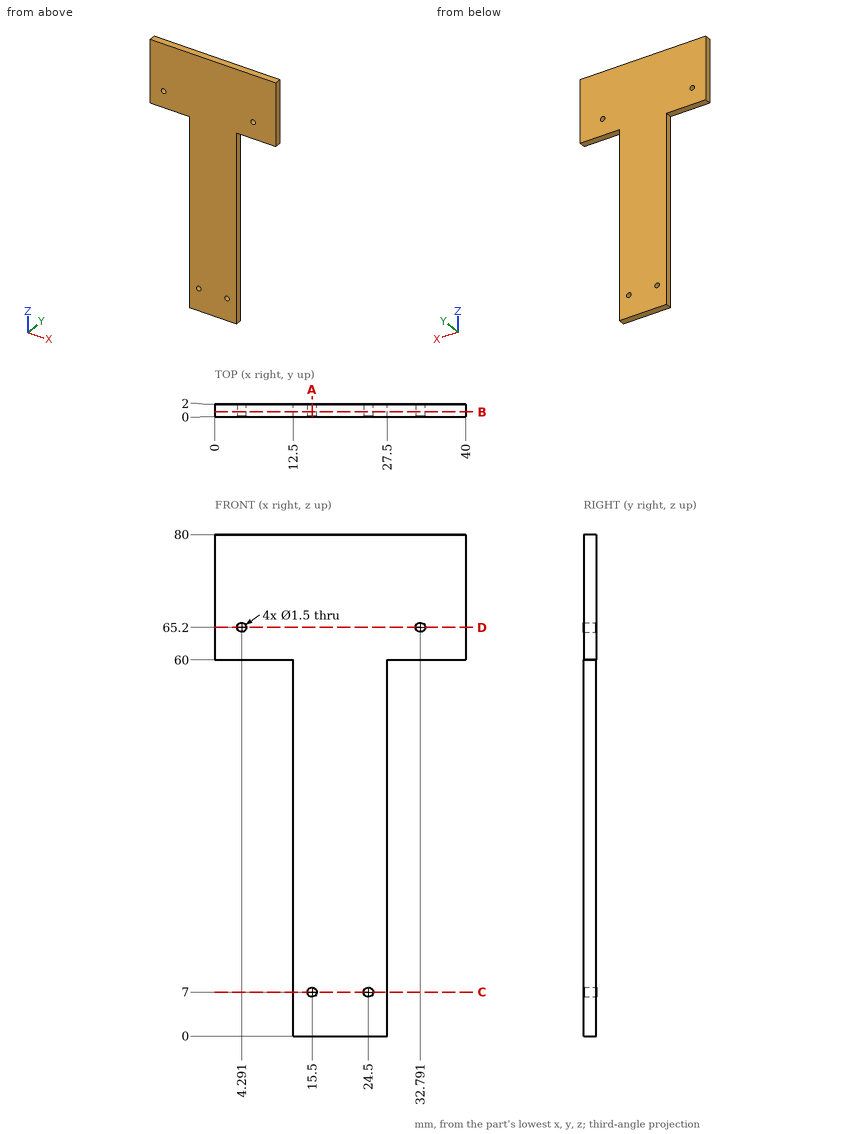
Geometry check sheet. Reference: drawing and pictorial views, mm from the part's lowest x, y, z. Give positions to 0.01 mm unless a question says otherwise; leave off trailing zeros. Order: outer loops, then holes, each group sorted by start corner. A loop starts at its lowest first (then second) coordinate and runs counter-clockwise, first axis right, second up.
1. Section check C-C, the plane z = 7. Enter the section's corners in (x, y).
2. Section check B-B, the plane y = 0.75. Enter the section's corners in (x, z).
3. Gauge pin test, flat ends, axial feed: pin 1 Ø1.2 at (x, z) = (4.29, 65.2) entering from +Y; pin 2 Ø1 at (y, z) = (0.5, 51) entering from +X; pin 3 Ø1.7 at (x, z) = (32.79, 65.2) entering from -Y. Record the tip position at first contact, or that the pin passes through.
4. Thickness scan on L1, parallel to X at y = 1, z = 65.2; L2, parallel to Z at x = 15.5, y = 0.75; L3, parallel to Z at x = 31.5, y = 0.9. Record the ranges inside material, lowest first.
5. Section check D-D, the plane z = 65.2. Enter the section's corners in (x, y).
6. Section check A-A, the plane x = 15.5. Enter the section's corners in (y, z), and give its area (3 significant figures).
Values follow:
1. outline: (12.5, 0) - (14.75, 0) - (14.75, 2) - (12.5, 2) - close; (16.25, 0) - (23.75, 0) - (23.75, 2) - (16.25, 2) - close; (25.25, 0) - (27.5, 0) - (27.5, 2) - (25.25, 2) - close
2. outline: (0, 60) - (12.5, 60) - (12.5, 0) - (27.5, 0) - (27.5, 60) - (40, 60) - (40, 80) - (0, 80) - close; hole circle Ø1.5 at (4.29, 65.2); hole circle Ø1.5 at (15.5, 7); hole circle Ø1.5 at (24.5, 7); hole circle Ø1.5 at (32.79, 65.2)
3. pin 1: passes through
3. pin 2: stops at x = 27.5
3. pin 3: stops at y = 0
4. L1: x = 0 to 3.54, 5.04 to 32.04, 33.54 to 40
4. L2: z = 0 to 6.25, 7.75 to 80
4. L3: z = 60 to 80
5. outline: (0, 0) - (3.54, 0) - (3.54, 2) - (0, 2) - close; (5.04, 0) - (32.04, 0) - (32.04, 2) - (5.04, 2) - close; (33.54, 0) - (40, 0) - (40, 2) - (33.54, 2) - close
6. outline: (0, 0) - (2, 0) - (2, 6.25) - (0, 6.25) - close; (0, 7.75) - (2, 7.75) - (2, 80) - (0, 80) - close
6. area: 157 mm2
